Design review of the part built by this model. Coordinates are the model's own, in mm. A direction names the side the tool comes from. Coordinates: 2 decimals unless noted, no trailing zeros. Write each loop counter-clockwise with the first axis right and the second up, starting at its lowest first coordinate (ties: lowest second). Pieces come first, ordered by that corner, then holes.
Q1. To check wall thickness, follow probe 1 along Z at (x, y) = (47, -10); probe 2 along X at (y, z) = (-5.25, -67); probe 3 along X at (y, z) = (-5.5, -71). State the ranges of each line that lie inside material, in increasing order.
Q2. Add section A-A, the plane z = -66. Give the boundary of the cut face in (x, y).
Q3. Add section B-B, the plane x = 43. Give the boundary of the cut face in (y, z).
Q4. Machinability: for faces 1 (the face through (85, -8, 70)), 2 (the face through (66.517, -10.164, -105.341)), which of the approach directions +Z, -Z, +X, -X, +Y, -Y give a long, thin tool a straight path to every point of the face, cutting with its end or side? Answer none if there is none.
Q5. Clearance check with flat-ended pins moving along their axes: pin 1 Ø8 at (y, z) = (-10.5, -89) entering from -X; pin 2 Ø1.5 at (x, y) = (45, -14.5) entering from -Z; pin 3 Ø1.5 at (x, z) = (73, 57) entering from +Y. State where each tip first meets the part, or that it passes through.
from build123d import *

# Parameters (mm, degrees)
F0_W     = 85
F0_H     = 141.1
F1_DEPTH = 17
F2_R     = 4
F3_DEPTH = 77
F4_R     = 4
F5_DEPTH = 55.9
F5_TAPER = 0.5
F6_R     = 3.5121680905
F7_DEPTH = 30
F7_TAPER = 6


with BuildPart() as f1:
    # F0 (on Front) → F1 (new body)
    with BuildSketch(Plane.XZ):
        with Locations((42.5, 70.55)):
            Rectangle(F0_W, F0_H)
    extrude(amount=F1_DEPTH)

    # F2 (on face) → F3 (join)
    with BuildSketch(Plane(origin=(0, 0, 0), x_dir=(1, 0, 0), z_dir=(0, 0, -1))):
        with Locations((64.5, 7)):
            Circle(F2_R)
    extrude(amount=F3_DEPTH)

    # F4 (on face) → F5 (join)
    with BuildSketch(Plane(origin=(0, 0, -77), x_dir=(1, 0, 0), z_dir=(0, 0, -1))):
        with Locations((64.5, 7)):
            Circle(F4_R)
    extrude(amount=F5_DEPTH, taper=F5_TAPER)

    # F6 (on face) → F7 (join)
    with BuildSketch(Plane(origin=(0, 0, -132.9), x_dir=(1, 0, 0), z_dir=(0, 0, -1))):
        with Locations((64.5, 7)):
            Circle(F6_R)
    extrude(amount=F7_DEPTH, taper=F7_TAPER)


solid = f1.part
Here are the results:
1. probe 1: z = 0 to 141.1
1. probe 2: x = 60.9 to 68.1
1. probe 3: x = 60.79 to 68.21
2. outline: circle Ø8 at (64.5, -7)
3. outline: (-17, 0) - (0, 0) - (0, 141.1) - (-17, 141.1) - close
4. face 1: +Z, -Z, +X, +Y, -Y
4. face 2: -Z
5. pin 1: stops at x = 60.59
5. pin 2: stops at z = 0
5. pin 3: stops at y = 0
